Model file for the job. Use its own axes, mm. A direction names the side the tool comes from. Give positions to 0.01 mm unless a question says otherwise; leave off trailing zeros. Write each loop counter-clockwise with the first axis right and the second up, starting at its lowest first coordinate (ties: lowest second). Pieces come first, ordered by that corner, then holes. Notation, with made-up numbers: (-28, -28.75) - (2, -28.75) arc R19 cw to (2, -15.75) - close; hole circle Ø5 at (-8.75, 70). An arc over 180 degrees is marked (long way). Use CSV: the item, a comma, the result in double quotes.
Autodesk Inventor part; units mm, degrees
ref_plane "Start Plane" through (0, 0, 0) normal (0, 0, 1) x (1, 0, 0)
ref_plane "End Plane" through (0, 0, 2064.7518) normal (0, 0, 1) x (1, 0, 0)
ref_plane "Work Plane4" through (0, -20, 0) normal (0, 0.3827, -0.9239) x (1, 0, 0)
ref_plane "Start Plane" through (0, 0, 0) normal (0, 0, 1) x (1, 0, 0)
ref_plane "End Plane" through (0, 0, 2064.7518) normal (0, 0, 1) x (1, 0, 0)
sketch "Sketch" plane through (0, 0, 0) normal (0, 0, 1) x (1, 0, 0)
  line L0 (-20, -16) -> (-20, 16)
  line L1 (-16, 20) -> (16, 20)
  line L2 (20, 16) -> (20, -16)
  line L3 (16, -20) -> (-16, -20)
  arc A0 (-20, -16) -> (-16, -20) centre (-16, -16) ccw
  arc A1 (20, 16) -> (16, 20) centre (16, 16) ccw
  arc A2 (-16, 20) -> (-20, 16) centre (-16, 16) ccw
  arc A3 (16, -20) -> (20, -16) centre (16, -16) ccw
  arc A4 (-16, 18) -> (-18, 16) centre (-16, 16) ccw
  line L4 (-16, 18) -> (16, 18)
  arc A5 (18, 16) -> (16, 18) centre (16, 16) ccw
  line L5 (18, 16) -> (18, -16)
  arc A6 (16, -18) -> (18, -16) centre (16, -16) ccw
  line L6 (16, -18) -> (-16, -18)
  arc A7 (-18, -16) -> (-16, -18) centre (-16, -16) ccw
  line L7 (-18, -16) -> (-18, 16)
  line L8 (0, 29.1598) -> (0, -29.1598) construction
  line L9 (-29.1598, 0) -> (29.1598, 0) construction
  dimension "d7" = 4
  dimension "d9" = 40
  dimension "d11" = 40
  dimension "d12" = 2
  dimension "d15" = 20
  dimension "d16" = 20
extrude "Body" add sketch "Sketch" along normal up to surface (2064.7518 mm away) from surface at 0
sketch "Sketch3" plane through (0, 0, 0) normal (0, 0, 1) x (1, 0, 0)
  line L0 (0, 0) -> (10, 0)
ref_plane "Work Plane3" through (0, 0, 0) normal (0, -1, 0) x (1, 0, 0)
ref_plane "Work Plane4" through (0, -20, 0) normal (0, 0.3827, -0.9239) x (1, 0, 0)
split "Split1" plane through (0, -20, 0) removes the side toward (0, 0.3827, -0.9239)
ref_plane "Work Plane5" through (16, 1323.5029, 721.2489) normal (0, 0.7071, 0.7071) x (1, 0, 0)
split "Split2" plane through (16, 1323.5029, 721.2489) removes the side toward (0, 0.7071, 0.7071)
sketch "Sketch4" plane through (0, 0, 0) normal (0, -1, 0) x (1, 0, 0)
  line L0 (-2, 0) -> (12, 0)
  line L1 (-2, 2064.7518) -> (12, 2064.7518)
  dimension "d18" = 2064.7518
equation "\"d7\" = G_IR"
equation "\"d9\" = G_W"
equation "\"d11\" = G_H"
equation "\"d12\" = G_T"
equation "\"d15\" = 0.5 * d9"
equation "\"d16\" = 0.5 * d11"
equation "\"d3\" = G_L"
equation "\"G_W\" = 40"
equation "\"G_H\" = 40"
equation "\"G_T\" = 2"
equation "\"G_IR\" = 4"
equation "\"G_L\" = d18"
equation "\"G_OFFSET_START\" = 0"
equation "\"G_OFFSET_END\" = -56.56854"
equation "\"d14\" = G_OFFSET_END + B_L"
equation "\"B_L\" = 2121.32034"
properties part number "ISO 10799-2 - 40x40x2 - 2064,75" material "Stainless Steel"
(1) 3-axis set-ups, long thin cutter, end or side, ignore diameter. For faces 4 (the face through (18, 0, 1017)), 5 (the face through (0, 20, 1007)): which of +Z, -Z, +X, -X, +Y, -Y reach the whole face in a straight line?
Checked values:
face 4,"+Z, -Z"
face 5,"+Z, -Z, +X, -X, +Y"
(2) Flat gauge pins, fed straight in: P1, Ø12, axis at x = 14, y = 3.5, coming from the -Z side; P2, Ø12, axis at x = 14.5, y = -1, coming from the +Z side. Where does each tip first touch, or does it go through?
Checked values:
P1,"stops at z = 7.88"
P2,"stops at z = 2050.63"
(3) Pull direction X, two halves, no side cores. Call faces 1 (the face through (0, -18, 1017)), 2 (the face through (20, 0, 1017)), 3 (the face through (0, -20, 1018)): released by +X, released by -X, zero draft, split by the parting line, or undercut.
Checked values:
face 1,"undercut"
face 2,"released by +X"
face 3,"zero draft"
(4) Wall check: probe 1 along X at (y, z) = (17, 350); probe 2 along Y at (x, z) = (-12.5, 445). Give the ranges that are in metal, low to high. Write a range as [from, to].
Checked values:
probe 1,"x = [-19.87, -17.73], [17.73, 19.87]"
probe 2,"y = [-20, -18], [18, 20]"
(5) Saw through at B-B, the plane z = 1679.5. List the corners of the cut face in (x, y), then the cut area to 3 significant figures.
Checked values:
outline,"(-20, -16) arc R4 ccw to (-16, -20) - (16, -20) arc R4 ccw to (20, -16) - (20, 16) arc R4 ccw to (16, 20) - (-16, 20) arc R4 ccw to (-20, 16) - close; hole (-18, -16) arc R2 ccw to (-16, -18) - (16, -18) arc R2 ccw to (18, -16) - (18, 16) arc R2 ccw to (16, 18) - (-16, 18) arc R2 ccw to (-18, 16) - close"
area,"294 mm^2"
(6) Saw through at A-A, the plane x = -0.5. List the corners of the cut face in (y, z).
Checked values:
outline,"(-20, 0) - (-18, 0.83) - (-18, 2062.75) - (-20, 2064.75) - close; (18, 15.74) - (20, 16.57) - (20, 2024.75) - (18, 2026.75) - close"
(7) Saw through at C-C, the plane y = 1.5. List the corners of the cut face in (x, z), then the cut area to 3 significant figures.
Checked values:
outline,"(-20, 8.91) - (-18, 8.91) - (-18, 2043.25) - (-20, 2043.25) - close; (18, 8.91) - (20, 8.91) - (20, 2043.25) - (18, 2043.25) - close"
area,"8,140 mm^2"
